Verification items for the finished model (mm, model axes). Coordinates: 2 decimals unless noted, no trailing zeros. Write each loop counter-clockwise with the first axis right and the second up, starting at its lowest first coordinate (ties: lowest second). Pieces come first, ordered by that corner, then holes. Notation, with made-up numbers: (60.5, 71.5) - (89.5, 71.5) arc R31 cw to (89.5, 98.5) - close; hole circle Ø2 at (-38, 17). An arc over 180 degrees is marked (long way). Use one line per item in the form item = value. Start each with the question number.
(1) Sectioned sample at D-D (y = 9). Record the cut outline in (x, z), and give its area (3 significant figures).
(2) Gauge pin test, flat ends, axial feed: pin 1 Ø10 at (y, z) = (25.5, -8) entering from -X; pin 2 Ø10 at (x, z) = (10, 5) entering from -Y; pin 3 Ø3 at (x, z) = (3.5, 7) entering from -Y. Record the tip position at first contact, or that the pin passes through.
(3) Sectioned sample at A-A (y = 15.75). Record the cut outline in (x, z).
(4) Material ranges on line 1 (Z direction, x = 0, y = 13.25); line 2 (X direction, y = 19.25, z = 0.25); line 3 (Z direction, x = 0, y = 9.75), recorded low to high. Write a range as [from, to].
(5) Sectioned sample at C-C (z = 9.5). Record the cut outline in (x, y).
(6) Sectioned sample at B-B (x = 11.5). Record the cut outline in (y, z), and give its area (3 significant figures).
Autodesk Inventor part; units mm, degrees
ref_plane "YZ Plane" through (0, 0, 0) normal (1, 0, 0) x (0, 1, 0)
ref_plane "XZ Plane" through (0, 0, 0) normal (0, 1, 0) x (-1, 0, 0)
ref_plane "XY Plane" through (0, 0, 0) normal (0, 0, 1) x (1, 0, 0)
sketch "Эскиз1" plane through (0, 0, 0) normal (0, 0, 1) x (1, 0, 0)
  arc A0 (0, 0) -> (0, 30) centre (0, 15) ccw
  line L0 (0, 0) -> (0, 30)
  dimension "d0" = 30
revolve "Вращение1" add sketch "Эскиз1" angle 360 about axis through (0, 0, 0) along (0, 1, 0)
sketch "Эскиз2" plane through (0, 0, 0) normal (0, 1, 0) x (-1, 0, 0)
  point P0 (0, 0)
  point P1 (0, 0)
hole "Отверстие1" at (0, 0, 0) direction (0, 1, 0) diameter 8.376 depth 18 tip angle 118 counterbore diameter 12 counterbore depth 4
chamfer "Фаска1" distance 1.6 angle 45 1 edges at (0, 4, 4.188)
properties part number "Ручка"
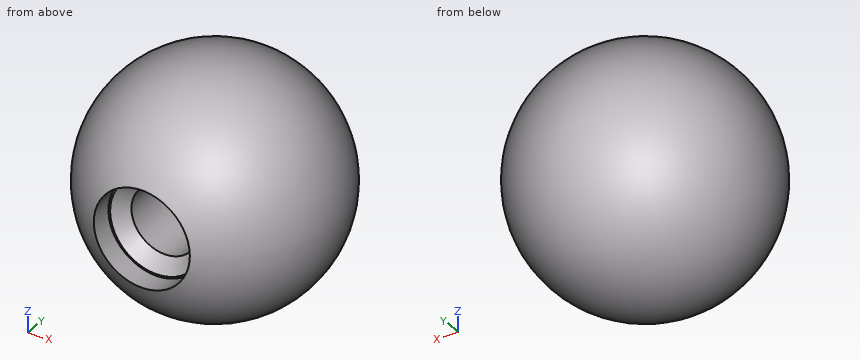
Answers below:
q1.outline = circle Ø27.5 at (0, 0); hole circle Ø8.38 at (0, 0)
q1.area = 539 mm2
q2.pin_1 = -12.56
q2.pin_2 = 1.33
q2.pin_3 = 1.4
q3.outline = circle Ø29.96 at (0, 0); hole circle Ø8.38 at (0, 0)
q4.line_1 = [-14.9, -4.19], [4.19, 14.9]
q4.line_2 = [-14.38, -2.09], [2.09, 14.38]
q4.line_3 = [-14.05, -4.19], [4.19, 14.05]
q5.outline = circle Ø23.22 at (0, 15)
q6.outline = circle Ø19.26 at (15, 0)
q6.area = 291 mm2
